For this review, take the finished solid that the model builds, in its own axes (mm). A direction names the side the tool comes from. Round coordinates to 2 decimals unless told otherwise and drop trailing zeros. Loops run counter-clockwise (first coordinate to the right, second up) from the corner with the lowest first, then second, coordinate; pieces in that order, holes last.
1) Take a section at B-B (z = 9). State the section outline as (x, y) points.
2) Insertion check: pin 1 (5 mm diameter, centred on y = 15.5, z = 11, fed in from -X); pin 2 (12 mm diameter, centred on y = 10.5, z = -8, fed in from +X); pin 3 (5.5 mm diameter, centred on x = 0.5, y = 26.5, fed in from +Z). Each pin has a flat end and moves straight along its axis. Give the tip position at first contact, or say it passes through.
3) Mouldability with a two-part tool opening along Z and no side actions: class faces 6 (the flat face through (22, 2, -22.669)), 7 (the flat face through (-22, 2, 14.669)), 8 (the flat face through (-22, 0, -19)), 9 (the flat face through (-18.09, 15.14, 12.3)) as pulls with the +Z half, pulls with the -Z half, needs draft (parallel to the pull), parting line crosses it, or undercut.
4) Take a section at D-D (x = -19.5). State the section outline as (y, z) points, then the cut area to 3 significant figures.
5) Wall thickness on L1, parallel to X at y = 21.5, z = 11; L2, parallel to Y at x = 25, z = 17.5; L3, parallel to Z at x = 10, y = 28.75: over which ranges is each line inside the solid? List them lowest first.
6) Take a section at A-A (z = 0). State the section outline as (x, y) points, then the cut area to 3 significant figures.
7) Tool access review of faces 1 (the flat face through (-18.09, 15.14, -12.3)), 2 (the flat face through (15.622, 15, 15)), 3 (the flat face through (23, 5, 20.4)), 4 (the flat face through (-20.622, 26, 0)), 5 (the flat face through (-15.622, 15, -15)): name each direction out of +Z, -Z, +X, -X, +Y, -Y from which nothing blocks a thin tool from reaching the whole face with its end or side.
8) Take a section at C-C (x = 10). State the section outline as (y, z) points.
```python
from build123d import *

# Parameters (mm, degrees)
SKETCH_1_W               = 12
SKETCH_1_H               = 8
SKETCH_1_R               = 1.5
EXTRUDE_1_DEPTH          = 5
EXTRUDE_2_DEPTH          = 5
SKETCH_3_W               = 15.622
SKETCH_3_H               = 15
SKETCH_3_R               = 2.5
EXTRUDE_3_DEPTH          = 5
MIRROR_5_COPY_1_SKETCH_W = 12
MIRROR_5_COPY_1_SKETCH_H = 8
MIRROR_5_COPY_1_SKETCH_R = 1.5
MIRROR_5_COPY_1_DEPTH    = 5
MIRROR_5_COPY_2_DEPTH    = 5


with BuildPart() as part:
    # Sketch 1 → Extrude 1 (new body)
    with BuildSketch(Plane(origin=(0, 0, 0), x_dir=(1, 0, 0), z_dir=(0, 1, 0))):
        with Locations((-21.622, -18.669)):
            Rectangle(SKETCH_1_W, SKETCH_1_H)
        with Locations(Location((-23.622, -18.669, 0), (0, 0, 270))):
            Circle(SKETCH_1_R, mode=Mode.SUBTRACT)
    extrude_1 = extrude(amount=EXTRUDE_1_DEPTH)

    # Sketch 2 → Extrude 2 (add)
    with BuildSketch(Plane(origin=(-15.622, 0, 0), x_dir=(0, 0, -1), z_dir=(1, 0, 0))):
        Polygon((-10, 25), (-14.669, 5), (-14.669, 0), (-19.669, 0), (-19.669, 5), (-13.83275, 30), (0, 30), (0, 25), align=None)
    extrude_2 = extrude(amount=-EXTRUDE_2_DEPTH)

    # Mirror 4: Extrude 1, Extrude 2 across plane
    add(extrude_1.mirror(Plane.XY))
    add(extrude_2.mirror(Plane.XY))

    # Sketch 3 → Extrude 3 (add)
    with BuildSketch(Plane(origin=(0, 30, 0), x_dir=(1, 0, 0), z_dir=(0, 1, 0))):
        with Locations((-7.811, 0)):
            Rectangle(SKETCH_3_W, SKETCH_3_H)
        with Locations(Location((-10, 0, 0), (0, 0, 270))):
            Circle(SKETCH_3_R, mode=Mode.SUBTRACT)
    extrude_3 = extrude(amount=-EXTRUDE_3_DEPTH)

    # Mirror 5: Extrude 1, Extrude 2, Extrude 3 across plane
    add(extrude_1.mirror(Plane(origin=(0, 0, 0), x_dir=(0, 0, 1), z_dir=(1, 0, 0))))
    add(extrude_2.mirror(Plane(origin=(0, 0, 0), x_dir=(0, 0, 1), z_dir=(1, 0, 0))))
    add(extrude_3.mirror(Plane(origin=(0, 0, 0), x_dir=(0, 0, 1), z_dir=(1, 0, 0))))



with BuildPart() as body_2:
    # Mirror 5 copy 1 sketch → Mirror 5 copy 1 (new body)
    with BuildSketch(Plane(origin=(0, 0, 0), x_dir=(-1, 0, 0), z_dir=(0, 1, 0))):
        with Locations((-21.622, -18.669)):
            Rectangle(MIRROR_5_COPY_1_SKETCH_W, MIRROR_5_COPY_1_SKETCH_H)
        with Locations(Location((-23.622, -18.669, 0), (0, 0, 270))):
            Circle(MIRROR_5_COPY_1_SKETCH_R, mode=Mode.SUBTRACT)
    extrude(amount=MIRROR_5_COPY_1_DEPTH)


with BuildPart() as part_1:
    add(part.part)

    add(body_2.part)  # Mirror 5 copy 2 merges body 2
    # Mirror 5 copy 2 sketch → Mirror 5 copy 2 (add)
    with BuildSketch(Plane.ZY.offset(-15.622)):
        Polygon((-10, 25), (-14.669, 5), (-14.669, 0), (-19.669, 0), (-19.669, 5), (-13.83275, 30), (0, 30), (0, 25), align=None)
    extrude(amount=-MIRROR_5_COPY_2_DEPTH)


solid = part_1.part
```
Response:
1. outline: (-20.62, 25) - (-15.62, 25) - (-15.62, 30) - (-20.62, 30) - close; (15.62, 25) - (20.62, 25) - (20.62, 30) - (15.62, 30) - close
2. pin 1: stops at x = -20.62
2. pin 2: stops at x = 20.62
2. pin 3: stops at z = 7.5
3. face 6: pulls with the -Z half
3. face 7: undercut
3. face 8: needs draft
3. face 9: undercut
4. outline: (0, -22.67) - (5, -22.67) - (5, -19.67) - (30, -13.83) - (30, 13.83) - (5, 19.67) - (5, 22.67) - (0, 22.67) - (0, 14.67) - (5, 14.67) - (25, 10) - (25, -10) - (5, -14.67) - (0, -14.67) - close
4. area: 424 mm2
5. L1: x = -20.62 to -15.62, 15.62 to 20.62
5. L2: y = 0 to 5
5. L3: z = -7.5 to -2.5, 2.5 to 7.5
6. outline: (-20.62, 25) - (-12.5, 25) - (-12.5, 30) - (-20.62, 30) - close; (-7.5, 25) - (7.5, 25) - (7.5, 30) - (-7.5, 30) - close; (12.5, 25) - (20.62, 25) - (20.62, 30) - (12.5, 30) - close
6. area: 156 mm2
7. face 1: +X, -X, -Y
7. face 2: +Z, +Y, -Y
7. face 3: +Z, +X, +Y
7. face 4: +Z, -Z, -X, +Y
7. face 5: -Z, +Y, -Y
8. outline: (25, -7.5) - (30, -7.5) - (30, -2.5) - (25, -2.5) - close; (25, 2.5) - (30, 2.5) - (30, 7.5) - (25, 7.5) - close
